```python
from build123d import *

# Parameters (mm, degrees)
BOSS_EXTRUDE1_DEPTH = 1168.4
CUT_EXTRUDE1_REACH  = 1170.87
SKETCH3_R           = 2.413
CUT_EXTRUDE2_REACH  = 1170.87
SKETCH4_R           = 2.413
LPATTERN1_COUNT     = 10
LPATTERN1_PITCH     = 114.3
SKETCH5_R           = 2.413
CUT_EXTRUDE3_DEPTH  = 1169.87011602
CUT_EXTRUDE4_REACH  = 1170.87
SKETCH6_R           = 2.413


with BuildPart() as part:
    # Sketch1 → Boss-Extrude1 (new body)
    with BuildSketch(Plane.XY):
        Polygon((3.175, 3.175), (3.175, 12.7), (0, 12.7), (0, 0), (31.75, 0), (31.75, 12.7), (28.575, 12.7), (28.575, 3.175), align=None)
    extrude(amount=BOSS_EXTRUDE1_DEPTH)

    # Sketch3 → Cut-Extrude1 (cut, up to next)
    with BuildSketch(Plane(origin=(0, 3.175, 0), x_dir=(1, 0, 0), z_dir=(0, 1, 0)), mode=Mode.PRIVATE) as cut_extrude1_sk1:
        with Locations(Location((11.1125, -1109.6625, 0), (0, 0, 270))):
            Circle(SKETCH3_R)
    cut_extrude1_tool1 = extrude(cut_extrude1_sk1.sketch, amount=-CUT_EXTRUDE1_REACH, mode=Mode.PRIVATE) & part.part
    # Sketch3 → Cut-Extrude1 (cut, up to next)
    with BuildSketch(Plane(origin=(0, 3.175, 0), x_dir=(1, 0, 0), z_dir=(0, 1, 0)), mode=Mode.PRIVATE) as cut_extrude1_sk2:
        with Locations(Location((20.6375, -1122.3625, 0), (0, 0, 270))):
            Circle(SKETCH3_R)
    cut_extrude1_tool2 = extrude(cut_extrude1_sk2.sketch, amount=-CUT_EXTRUDE1_REACH, mode=Mode.PRIVATE) & part.part
    cut_extrude1_1 = cut_extrude1_tool1.solids().sort_by_distance((11.1125, 3.175, 1109.6625))[0]
    add(cut_extrude1_1, mode=Mode.SUBTRACT)
    cut_extrude1_2 = cut_extrude1_tool2.solids().sort_by_distance((20.6375, 3.175, 1122.3625))[0]
    add(cut_extrude1_2, mode=Mode.SUBTRACT)
    cut_extrude1 = cut_extrude1_1 + cut_extrude1_2  # Cut-Extrude1 as one shape, for the pattern or mirror that repeats it

    # Sketch4 → Cut-Extrude2 (cut, up to next)
    with BuildSketch(Plane(origin=(0, 3.175, 0), x_dir=(1, 0, 0), z_dir=(0, 1, 0)), mode=Mode.PRIVATE) as cut_extrude2_sk1:
        with Locations(Location((15.875, -1158.875, 0), (0, 0, 270))):
            Circle(SKETCH4_R)
    cut_extrude2_tool1 = extrude(cut_extrude2_sk1.sketch, amount=-CUT_EXTRUDE2_REACH, mode=Mode.PRIVATE) & part.part
    add(cut_extrude2_tool1.solids().sort_by_distance((15.875, 3.175, 1158.875))[0], mode=Mode.SUBTRACT)

    # LPattern1: Cut-Extrude1 ×10
    with Locations(*[(0, 0, -i * LPATTERN1_PITCH) for i in range(1, LPATTERN1_COUNT)]):
        add(cut_extrude1, mode=Mode.SUBTRACT)

    # Sketch5 → Cut-Extrude3 (cut, through all)
    with BuildSketch(Plane(origin=(0, 3.175, 0), x_dir=(1, 0, 0), z_dir=(0, 1, 0))):
        with Locations(Location((20.6375, -46.0375, 0), (0, 0, 270))):
            Circle(SKETCH5_R)
        with Locations(Location((11.1125, -33.3375, 0), (0, 0, 270))):
            Circle(SKETCH5_R)
        with Locations((-236.5375, -33.3375)):
            Circle(SKETCH5_R)
        with Locations((-227.0125, -46.0375)):
            Circle(SKETCH5_R)
    extrude(amount=-CUT_EXTRUDE3_DEPTH, mode=Mode.SUBTRACT)

    # Sketch6 → Cut-Extrude4 (cut, up to next)
    with BuildSketch(Plane(origin=(0, 3.175, 0), x_dir=(1, 0, 0), z_dir=(0, 1, 0)), mode=Mode.PRIVATE) as cut_extrude4_sk1:
        with Locations(Location((15.875, -15.875, 0), (0, 0, 270))):
            Circle(SKETCH6_R)
    cut_extrude4_tool1 = extrude(cut_extrude4_sk1.sketch, amount=-CUT_EXTRUDE4_REACH, mode=Mode.PRIVATE) & part.part
    add(cut_extrude4_tool1.solids().sort_by_distance((15.875, 3.175, 15.875))[0], mode=Mode.SUBTRACT)


solid = part.part
```
Could you check a few things on this model? Use its own coordinates, in mm. A direction names the side the tool comes from. Round coordinates to 2 decimals unless told otherwise and drop trailing zeros. Loops run counter-clockwise (first coordinate to the right, second up) from the corner with the lowest first, then second, coordinate; pieces in that order, holes last. Notation, with made-up numbers: (57.25, -5.75) - (91.25, -5.75) arc R24 ccw to (91.25, 19.25) - close; hole circle Ø3 at (-33.5, 52.5). An arc over 180 degrees is marked (long way). Answer as CSV lines item,"result".
1. I want a section at B-B on z = 392. List the corners of the cut face in (x, y) for me (3 decimals), then the cut area to 3 significant figures.
Filled in:
outline,"(0, 0) - (31.75, 0) - (31.75, 12.7) - (28.575, 12.7) - (28.575, 3.175) - (3.175, 3.175) - (3.175, 12.7) - (0, 12.7) - close"
area,"161 mm^2"
2. For pin 1 Ø7.5 at (x, z) = (11.11, 195.26) entering from +Y (3 decimals), with a flat end and sliding along its axis, tell me the tip position at first contact or that it passes through.
Filled in:
pin 1,"stops at y = 3.175"
3. Please list where these lines run through material, in increasing order: line 1 along X through (y, z) = (3.75, 732.5) (3 decimals); line 2 along Y through (x, z) = (25, 898) (3 decimals). Write a range as [from, to].
Filled in:
line 1,"x = [0, 3.175], [28.575, 31.75]"
line 2,"y = [0, 3.175]"
4. I want a section at A-A on y = 10.25. List the corners of the cut face in (x, z) for me (3 decimals), then the cut area to 3 significant figures.
Filled in:
outline,"(0, 0) - (3.175, 0) - (3.175, 1168.4) - (0, 1168.4) - close; (28.575, 0) - (31.75, 0) - (31.75, 1168.4) - (28.575, 1168.4) - close"
area,"7,420 mm^2"
5. On a 3-axis mill with a long thin cutter (end or side, diameter ignored), from which of +Z, -Z, +X, -X, +Y, -Y can I reach the whole of each face in a straight line? I mean faces 1 (the face through (16, 0, 576)), 2 (the face through (16, 3.175, 576)). Say none if no direction works.
Filled in:
face 1,"+Z, -Z, +X, -X, -Y"
face 2,"+Z, -Z, +Y"
